Geometry: final body of the model. Coordinates: model frame, mm. A direction names the side the tool comes from. Coordinates: 2 decimals unless noted, no trailing zeros. Loops run counter-clockwise (first coordinate to the right, second up) from the corner with the lowest first, then second, coordinate; pieces in that order, holes last. Notation, with made-up numbers: (-36, 44) -> (-18, 44) arc R23 ccw to (-18, 70) -> close; hole circle Ø5 at (-1, 70). An arc over 180 degrees is marked (long way). One line per item, written item: value. Start each with the question number.
Item 1: Mould query, pull axis X, two halves, no side actions, for faces 1 (the cylindrical face through (-7.757, 5.685, 23.55)), 2 (the flat face through (30, 16.732, 6)), 3 (the flat face through (43, 10.382, 6)). Classes: +X half, -X half, draft (parallel to the pull), parting line (faces both ways), or undercut.
Item 2: Section query B-B on y = 2.75. Return loops of the section in (x, z).
Item 3: Ray query, probe 1 along Z at (x, y) = (34.5, -6.75); probe 2 along X at (y, z) = (7, 35.5); probe 3 along X at (y, z) = (1.5, 7). Return the intervals inside material, ascending. Write a range as from..to.
Item 4: Section query A-A on z = 5. Return loops of the section in (x, y), then the cut area to 3 significant figures.
Item 5: Set-up query: faces 4 (the flat face through (21, 4, 0)), 5 (the flat face through (5, 4, 12.7)), 6 (the cylindrical face through (23.887, 4.171, 6.439)). Return all of +Z, -Z, +X, -X, +Y, -Y with unobstructed straight access to the full face (end or side cutting, diameter ignored); none if empty.
Item 6: Section query D-D on x = 6. Return loops of the section in (y, z), then the cut area to 3 significant figures.
Item 7: Section query C-C on x = 26. Return loops of the section in (y, z), then the cut area to 3 significant figures.
Item 8: Contact query for flat-ended pins moving along their axis: pin 1 Ø7.5 at (x, y) = (4.84, 4.03) entering from +Z; pin 2 Ø10 at (y, z) = (8, 16.5) entering from +X (3 decimals); pin 3 Ø2 at (y, z) = (5, 13) entering from -X; pin 4 Ø10 at (y, z) = (7.5, 29.5) entering from +X. Output: stop coordinate, or through.
from build123d import *

# Parameters (mm, degrees)
F0_W      = 76.2
F0_H      = 25.4
F1_DEPTH  = 38.1
F2_W      = 50.8
F2_H      = 25.4
F3_DEPTH  = 25.4
F5_DEPTH  = 25.4
F7_DEPTH  = 25.4
F8_DEPTH  = 25.4
F10_DEPTH = 25.4
F12_DEPTH = 25.4


with BuildPart() as f1:
    # F0 (on Top) → F1 (new body)
    with BuildSketch(Plane.XY):
        with Locations((30.2353623112, 4.0315114893)):
            Rectangle(F0_W, F0_H)
    extrude(amount=F1_DEPTH)

    # F2 (on face) → F3 (cut)
    with BuildSketch(Plane.XZ.offset(8.6684885107)):
        with Locations((42.9353623112, 25.4)):
            Rectangle(F2_W, F2_H)
    extrude(amount=-F3_DEPTH, mode=Mode.SUBTRACT)

    # F4 (on face) → F5 (cut)
    with BuildSketch(Plane.XY.offset(38.1)):
        with BuildLine():
            ThreePointArc((11.1853623112, 4.0315114893), (4.8353623112, 10.3815114893), (-1.5146376888, 4.0315114893))
            Line((-1.5146376888, 4.0315114893), (11.1853623112, 4.0315114893))
        make_face()
        with BuildLine():
            Line((11.1853623112, 4.0315114893), (-1.5146376888, 4.0315114893))
            ThreePointArc((-1.5146376888, 4.0315114893), (4.8353623112, -2.3184885107), (11.1853623112, 4.0315114893))
        make_face()
    extrude(amount=-F5_DEPTH, mode=Mode.SUBTRACT)

    # F6 (on face) → F7 (cut)
    with BuildSketch(Plane.XY.offset(38.1)):
        with BuildLine():
            ThreePointArc((-7.8646376888, 4.0315114893), (-4.1448937926, 13.0117676276), (4.8353623599, 16.7315114893))
            Line((4.8353623599, 16.7315114893), (-7.8646376888, 16.7315114893))
            Line((-7.8646376888, 16.7315114893), (-7.8646376888, 4.0315114893))
        make_face()
        with BuildLine():
            Line((-7.8646376888, -8.6684885107), (4.8353623112, -8.6684885107))
            ThreePointArc((4.8353623112, -8.6684885107), (-4.1448938098, -4.9487446318), (-7.8646376888, 4.0315114893))
            Line((-7.8646376888, 4.0315114893), (-7.8646376888, -8.6684885107))
        make_face()
        with BuildLine():
            Line((17.5353623112, -8.6684885107), (17.5353623112, 4.0315114893))
            ThreePointArc((17.5353623112, 4.0315114893), (13.8156184323, -4.9487446318), (4.8353623112, -8.6684885107))
            Line((4.8353623112, -8.6684885107), (17.5353623112, -8.6684885107))
        make_face()
        with BuildLine():
            ThreePointArc((4.8353623599, 16.7315114893), (13.8156184495, 13.0117675932), (17.5353623112, 4.0315114893))
            Line((17.5353623112, 4.0315114893), (17.5353623112, 16.7315114893))
            Line((17.5353623112, 16.7315114893), (4.8353623599, 16.7315114893))
        make_face()
    extrude(amount=-F7_DEPTH, mode=Mode.SUBTRACT)

    # F8 (cut): faces of the model
    f8_faces = [f1.faces().sort_by_distance(p)[0] for p in [
        (-5.0278648642, 13.8947386647, 12.7),
        (-5.0278648642, -5.8317156861, 12.7),
    ]]
    extrude(f8_faces, amount=-F8_DEPTH, mode=Mode.SUBTRACT)

    # F9 (on face) → F10 (cut)
    with BuildSketch(Plane.XY.offset(12.7)):
        with BuildLine():
            Line((30.2353623112, -2.3184885107), (55.6353623112, -2.3184885107))
            ThreePointArc((55.6353623112, -2.3184885107), (61.9853623112, 4.0315114893), (55.6353623112, 10.3815114893))
            Line((55.6353623112, 10.3815114893), (30.2353623112, 10.3815114893))
            ThreePointArc((30.2353623112, 10.3815114893), (23.8853623112, 4.0315114893), (30.2353623112, -2.3184885107))
        make_face()
    extrude(amount=-F10_DEPTH, mode=Mode.SUBTRACT)

    # F11 (on face) → F12 (cut)
    with BuildSketch(Plane.XY.offset(12.7)):
        with BuildLine():
            ThreePointArc((55.6353623112, 16.7315114893), (64.6156184323, 13.0117676104), (68.3353623112, 4.0315114893))
            Line((68.3353623112, 4.0315114893), (68.3353623112, 16.7315114893))
            Line((68.3353623112, 16.7315114893), (55.6353623112, 16.7315114893))
        make_face()
        with BuildLine():
            Line((68.3353623112, -8.6684885107), (68.3353623112, 4.0315114893))
            ThreePointArc((68.3353623112, 4.0315114893), (64.6156183701, -4.948744694), (55.6353621352, -8.6684885107))
            Line((55.6353621352, -8.6684885107), (68.3353623112, -8.6684885107))
        make_face()
    extrude(amount=-F12_DEPTH, mode=Mode.SUBTRACT)


solid = f1.part
Reply:
1. face 1: parting line
1. face 2: draft
1. face 3: undercut
2. outline: (-7.8, 0) -> (24.02, 0) -> (24.02, 12.7) -> (17.47, 12.7) -> (17.47, 38.1) -> (11.05, 38.1) -> (11.05, 12.7) -> (-1.38, 12.7) -> (-1.38, 38.1) -> (-7.8, 38.1) -> close; (61.85, 0) -> (68.27, 0) -> (68.27, 12.7) -> (61.85, 12.7) -> close
3. probe 1: z = 0..12.7
3. probe 2: x = -7.51..-0.78, 10.45..17.18
3. probe 3: x = -7.61..24.41, 61.46..68.08
4. outline: (4.84, -8.67) -> (55.64, -8.67) arc R12.7 ccw to (55.64, 16.73) -> (4.84, 16.73) arc R12.7 ccw to start; hole (30.24, -2.32) -> (55.64, -2.32) arc R6.35 ccw to (55.64, 10.38) -> (30.24, 10.38) arc R6.35 ccw to start
4. area: 1,350 mm²
5. face 4: -Z, +X, -X, +Y, -Y
5. face 5: +Z
5. face 6: +Z, -Z
6. outline: (-8.67, 0) -> (16.73, 0) -> (16.73, 12.7) -> (16.68, 12.7) -> (16.68, 38.1) -> (10.27, 38.1) -> (10.27, 12.7) -> (-2.21, 12.7) -> (-2.21, 38.1) -> (-8.61, 38.1) -> (-8.61, 12.7) -> (-8.67, 12.7) -> close
6. area: 648 mm²
7. outline: (-8.67, 0) -> (-0.7, 0) -> (-0.7, 12.7) -> (-8.67, 12.7) -> close; (8.76, 0) -> (16.73, 0) -> (16.73, 12.7) -> (8.76, 12.7) -> close
7. area: 202 mm²
8. pin 1: stops at z = 12.7
8. pin 2: stops at x = 68.315
8. pin 3: stops at x = -7.86
8. pin 4: stops at x = 17.54
